Here's how the part is built. I have some questions about the finished solid (model axes, mm). A direction names the side the tool comes from. Coordinates: 2 decimals unless noted, no trailing zeros. Order: outer loops, then holes, each group sorted by start corner. A loop starts at its lowest first (then second) coordinate and runs counter-clockwise, first axis right, second up.
```python
from build123d import *

# Parameters (mm, degrees)
SKETCH1_W                                = 60
SKETCH1_H                                = 35.17
BOSS_EXTRUDE1_DEPTH                      = 2.5
SKETCH2_W                                = 16.25
SKETCH2_H                                = 2.75
BOSS_EXTRUDE2_DEPTH                      = 35.17
CUT_EXTRUDE1_DEPTH                       = 70.745905973
CUT_EXTRUDE2_DEPTH                       = 70.745905973
SKETCH5_R                                = 1.75
BOSS_EXTRUDE3_DEPTH                      = 1.85
TAP_DRILL_FOR_M2_5X0_45_TAP1_D           = 2.05
TAP_DRILL_FOR_M2_5X0_45_TAP1_DEPTH       = 4
TAP_DRILL_FOR_M2_5X0_45_TAP1_CSINK_D     = 2.1
TAP_DRILL_FOR_M2_5X0_45_TAP1_CSINK_ANGLE = 90
TAP_DRILL_FOR_M2_5X0_45_TAP1_TIP         = 0.615882135
SKETCH14_R                               = 2.85
SKETCH14_R_2                             = 2.35
CUT_EXTRUDE4_DEPTH                       = 0.5
SKETCH15_W                               = 4.66
SKETCH15_H                               = 2.5
SKETCH15_W_2                             = 0.34
CUT_EXTRUDE5_DEPTH                       = 70.683939326
SKETCH9_R                                = 1.58
CUT_EXTRUDE3_DEPTH                       = 70.453632014
M3_CLEARANCE_HOLE1_D                     = 3.4
SKETCH17_W                               = 7
SKETCH17_H                               = 2.5
BOSS_EXTRUDE4_DEPTH                      = 35.17
SKETCH18_W                               = 0.25
SKETCH18_H                               = 2.75
CUT_EXTRUDE6_DEPTH                       = 76.494417012


with BuildPart() as part:
    # Sketch1 → Boss-Extrude1 (new body)
    with BuildSketch(Plane(origin=(0, 0, 0), x_dir=(1, 0, 0), z_dir=(0, 1, 0))):
        with Locations((30, 17.585)):
            Rectangle(SKETCH1_W, SKETCH1_H)
    extrude(amount=BOSS_EXTRUDE1_DEPTH)

    # Sketch2 → Boss-Extrude2 (add, through all)
    with BuildSketch(Plane.XY):
        with Locations((30.125, -1.375)):
            Rectangle(SKETCH2_W, SKETCH2_H)
    extrude(amount=-BOSS_EXTRUDE2_DEPTH)

    # Sketch3 → Cut-Extrude1 (cut, through all)
    with BuildSketch(Plane.XZ.offset(2.75)):
        with BuildLine():
            Line((21.16, -31.92), (24, -31.92))
            ThreePointArc((24, -31.92), (24.707106781, -31.627106781), (25, -30.92))
            Line((25, -30.92), (25, -3.92))
            ThreePointArc((25, -3.92), (24.707106781, -3.212893219), (24, -2.92))
            Line((24, -2.92), (21.16, -2.92))
            ThreePointArc((21.16, -2.92), (20.452893219, -3.212893219), (20.16, -3.92))
            Line((20.16, -3.92), (20.16, -30.92))
            ThreePointArc((20.16, -30.92), (20.452893219, -31.627106781), (21.16, -31.92))
        make_face()
    extrude(amount=-CUT_EXTRUDE1_DEPTH, mode=Mode.SUBTRACT)

    # Sketch4 → Cut-Extrude2 (cut, through all)
    with BuildSketch(Plane(origin=(0, 2.5, 0), x_dir=(1, 0, 0), z_dir=(0, 1, 0))):
        with BuildLine():
            Line((32.7475, 2.92), (32.7475, 7.42))
            ThreePointArc((32.7475, 7.42), (33.260063133, 8.657436867), (34.4975, 9.17))
            Line((34.4975, 9.17), (34.9975, 9.17))
            ThreePointArc((34.9975, 9.17), (36.234936867, 8.657436867), (36.7475, 7.42))
            Line((36.7475, 7.42), (36.7475, 2.92))
            ThreePointArc((36.7475, 2.92), (36.234936867, 1.682563133), (34.9975, 1.17))
            Line((34.9975, 1.17), (34.4975, 1.17))
            ThreePointArc((34.4975, 1.17), (33.260063133, 1.682563133), (32.7475, 2.92))
        make_face()
        with BuildLine():
            Line((32.7475, 28.42), (32.7475, 23.92))
            ThreePointArc((32.7475, 23.92), (33.260063133, 22.682563133), (34.4975, 22.17))
            Line((34.4975, 22.17), (34.9975, 22.17))
            ThreePointArc((34.9975, 22.17), (36.234936867, 22.682563133), (36.7475, 23.92))
            Line((36.7475, 23.92), (36.7475, 28.42))
            ThreePointArc((36.7475, 28.42), (36.234936867, 29.657436867), (34.9975, 30.17))
            Line((34.9975, 30.17), (34.4975, 30.17))
            ThreePointArc((34.4975, 30.17), (33.260063133, 29.657436867), (32.7475, 28.42))
        make_face()
    extrude(amount=-CUT_EXTRUDE2_DEPTH, mode=Mode.SUBTRACT)

    # Sketch5 → Boss-Extrude3 (add)
    with BuildSketch(Plane(origin=(0, 2.5, 0), x_dir=(1, 0, 0), z_dir=(0, 1, 0))):
        with Locations(Location((34.7475, 15.17, 0), (0, 0, 90))):
            Circle(SKETCH5_R)
    extrude(amount=BOSS_EXTRUDE3_DEPTH)

    # Tap Drill for M2.5x0.45 Tap1
    with Locations(Plane(origin=(0, 4.35, 0), x_dir=(1, 0, 0), z_dir=(0, 1, 0))):
        with Locations((34.7475, 15.17)):
            CounterSinkHole(TAP_DRILL_FOR_M2_5X0_45_TAP1_D / 2, TAP_DRILL_FOR_M2_5X0_45_TAP1_CSINK_D / 2, depth=TAP_DRILL_FOR_M2_5X0_45_TAP1_DEPTH, counter_sink_angle=TAP_DRILL_FOR_M2_5X0_45_TAP1_CSINK_ANGLE)
            with Locations((0, 0, -(TAP_DRILL_FOR_M2_5X0_45_TAP1_DEPTH + TAP_DRILL_FOR_M2_5X0_45_TAP1_TIP / 2))):  # 118° drill point
                Cone(0, TAP_DRILL_FOR_M2_5X0_45_TAP1_D / 2, TAP_DRILL_FOR_M2_5X0_45_TAP1_TIP, mode=Mode.SUBTRACT)

    # Sketch14 → Cut-Extrude4 (cut)
    with BuildSketch(Plane.XZ.offset(2.75)):
        with Locations((28.5, -25.31)):
            Circle(SKETCH14_R)
        with Locations((34.5, -18.31)):
            Circle(SKETCH14_R)
        with Locations((31, -11.31)):
            Circle(SKETCH14_R)
        with Locations((29, -4.31)):
            Circle(SKETCH14_R)
        with Locations((32.18, -32.31)):
            Circle(SKETCH14_R_2)
    extrude(amount=-CUT_EXTRUDE4_DEPTH, mode=Mode.SUBTRACT)

    # Sketch15 → Cut-Extrude5 (cut, through all)
    with BuildSketch(Plane(origin=(0, 0, -35.17), x_dir=(-1, 0, 0), z_dir=(0, 0, -1))):
        with Locations((-2.33, 1.25)):
            Rectangle(SKETCH15_W, SKETCH15_H)
        with Locations((-59.83, 1.25)):
            Rectangle(SKETCH15_W_2, SKETCH15_H)
    extrude(amount=-CUT_EXTRUDE5_DEPTH, mode=Mode.SUBTRACT)

    # Sketch9 → Cut-Extrude3 (cut, through all)
    with BuildSketch(Plane(origin=(0, 2.5, 0), x_dir=(1, 0, 0), z_dir=(0, 1, 0))):
        with Locations(Location((15.66, 17.5, 0), (0, 0, 270))):
            Circle(SKETCH9_R)
        with Locations(Location((48.66, 17.5, 0), (0, 0, 270))):
            Circle(SKETCH9_R)
    extrude(amount=-CUT_EXTRUDE3_DEPTH, mode=Mode.SUBTRACT)

    # M3 Clearance Hole1 (through all)
    with Locations(Plane(origin=(0, 2.5, 0), x_dir=(1, 0, 0), z_dir=(0, 1, 0))):
        with Locations((13.16, 7.5), (13.16, 27.5), (51.16, 27.5), (51.16, 7.5)):
            Hole(M3_CLEARANCE_HOLE1_D / 2)

    # Sketch17 → Boss-Extrude4 (add)
    with BuildSketch(Plane.XY):
        with Locations((63.16, 1.25)):
            Rectangle(SKETCH17_W, SKETCH17_H)
        with Locations((1.16, 1.25)):
            Rectangle(SKETCH17_W, SKETCH17_H)
    extrude(amount=-BOSS_EXTRUDE4_DEPTH)

    # Sketch18 → Cut-Extrude6 (cut, through all)
    with BuildSketch(Plane.XY):
        with Locations((38.125, -1.375)):
            Rectangle(SKETCH18_W, SKETCH18_H)
        with Locations((22.125, -1.375)):
            Rectangle(SKETCH18_W, SKETCH18_H)
    extrude(amount=-CUT_EXTRUDE6_DEPTH, mode=Mode.SUBTRACT)


solid = part.part
```
Q1. We'd pull the mould along X, two halves only. Please class faces 1 (the flat face through (22.25, -1, -1)), 2 (the cylindrical face through (33.27, -0.09, -29.67)), 3 (the flat face through (32, 1, -35.17)): pulls with the +X half, pulls with the -X half, needs draft (parallel to the pull), parting line crosses it, or undercut.
Q2. If we section it at B-B on z = -27.5: Write out the boundary of the cut face in (x, y).
Q3. For faces 4 (the cylindrical face through (34.67, 3.41, -13.42)), 5 (the flat face through (32.748, 0, -26)), 6 (the flat face through (10, 0, -17)), 7 (the flat face through (32, -2.25, -32)), 8 (the flat face through (66.66, 1, -17)), which set-ups out of +Z, -Z, +X, -X, +Y, -Y let a thin tool reach every point of the face, with its end or its side?
Q4. If we section it at A-A on x = 13.16: Write out the boundary of the cut face in (y, z), then the cut area to 3 significant figures.
Q5. I need wall thicknesses on L1, parallel to X at y = 0.7, z = -27.5; L2, parallel to Z at x = 51.16, y = 1.1; L3, parallel to X at y = 1.3, z = -17.5. Which ranges of each line are inside material? Lowest first, please.
Q6. If we section it at D-D on y = 1: Give the number of separate pieces and of enclosed holes in the cut face, then the cut area to 3 significant figures.
Q7. If we section it at C-C on x = 56: Write out the boundary of the cut face in (y, z), then the cut area to 3 significant figures.
Q8. Will these pins go through, and if not, where does the flat tip stop? pin 1 (1 mm diameter, centred on x = 23, y = 1, fed in from +Z); pin 2 (5 mm diameter, centred on x = 52.5, z = -28.5, fed in from -Y); pin 3 (4.5 mm diameter, centred on x = 31, z = -11.31, fed in from +Y); pin 4 (1.2 mm diameter, centred on x = 34.75, z = -15.17, fed in from +Y).
Reply:
1. face 1: pulls with the -X half
1. face 2: undercut
1. face 3: needs draft
2. outline: (-2.34, 0) - (11.46, 0) - (11.46, 2.5) - (-2.34, 2.5) - close; (14.86, 0) - (20.16, 0) - (20.16, 2.5) - (14.86, 2.5) - close; (25, -2.75) - (26.68, -2.75) - (26.68, -2.25) - (30.32, -2.25) - (30.32, -2.75) - (32.75, -2.75) - (32.75, 2.5) - (25, 2.5) - close; (36.75, -2.75) - (38, -2.75) - (38, 0) - (49.46, 0) - (49.46, 2.5) - (36.75, 2.5) - close; (52.86, 0) - (66.66, 0) - (66.66, 2.5) - (52.86, 2.5) - close
3. face 4: +Y
3. face 5: +Y, -Y
3. face 6: +Z, -Z, -X, -Y
3. face 7: -Y
3. face 8: +Z, -Z, +X, +Y, -Y
4. outline: (0, -35.17) - (2.5, -35.17) - (2.5, -29.2) - (0, -29.2) - close; (0, -25.8) - (2.5, -25.8) - (2.5, -9.2) - (0, -9.2) - close; (0, -5.8) - (2.5, -5.8) - (2.5, 0) - (0, 0) - close
4. area: 70.9 mm2
5. L1: x = -2.34 to 11.46, 14.86 to 20.16, 25 to 32.75, 36.75 to 49.46, 52.86 to 66.66
5. L2: z = -35.17 to -29.2, -25.8 to -9.2, -5.8 to 0
5. L3: x = -2.34 to 14.08, 17.24 to 20.16, 25 to 47.08, 50.24 to 66.66
6. separate pieces: 1
6. enclosed holes: 10
6. area: 2,170 mm2
7. outline: (0, -35.17) - (2.5, -35.17) - (2.5, 0) - (0, 0) - close
7. area: 87.9 mm2
8. pin 1: stops at z = 0
8. pin 2: stops at y = 0
8. pin 3: stops at y = 2.5
8. pin 4: stops at y = 0.1
